Could you check a few things on this model? Use its own coordinates, in mm. A direction names the side the tool comes from. Coordinates: 2 decimals unless noted, no trailing zeros. Order: outer loops, then holes, each group sorted by start corner. A loop starts at its lowest first (then second) coordinate and runs counter-clockwise, first axis right, second up. Notation, with made-up numbers: M 54,-22.75 L 112,-22.75 A23 cw 112,-4.75 Z; hole C 41,17.5 d6. An arc over 180 degrees is marked long. Write item = value, one per line. Start each with the question number.
from build123d import *

# Parameters (mm, degrees)
RESSALTO_EXTRUS_O1_DEPTH          = 10
REBAIXO_PARA_SHCS_M31_D           = 3.4
REBAIXO_PARA_SHCS_M31_CBORE_D     = 6.5
REBAIXO_PARA_SHCS_M31_CBORE_DEPTH = 3
ESBO_O5_W                         = 20.2
ESBO_O5_H                         = 10.9
CORTE_EXTRUS_O1_DEPTH             = 73.325928961
FILETE1_R                         = 5
FILETE2_R                         = 2


with BuildPart() as part:
    # Esboço1 → Ressalto-extrusão1 (new body)
    with BuildSketch(Plane(origin=(0, 0, 0), x_dir=(0, 0, -1), z_dir=(1, 0, 0))):
        Polygon((0, 0), (0, 6), (19.9, 6), (19.9, 15.2), (50.1, 15.2), (50.1, 6), (70, 6), (70, 0), align=None)
    extrude(amount=RESSALTO_EXTRUS_O1_DEPTH)

    # Rebaixo para SHCS M31 (through all)
    with Locations(Plane(origin=(0, 6, 0), x_dir=(1, 0, 0), z_dir=(0, 1, 0))):
        with Locations((5, 5), (5, 65)):
            CounterBoreHole(REBAIXO_PARA_SHCS_M31_D / 2, REBAIXO_PARA_SHCS_M31_CBORE_D / 2, REBAIXO_PARA_SHCS_M31_CBORE_DEPTH)

    # Esboço5 → Corte-extrusão1 (cut, through all)
    with BuildSketch(Plane(origin=(10, 0, 0), x_dir=(0, 0, -1), z_dir=(1, 0, 0))):
        with Locations((35, 5.45)):
            Rectangle(ESBO_O5_W, ESBO_O5_H)
    extrude(amount=-CORTE_EXTRUS_O1_DEPTH, mode=Mode.SUBTRACT)

    # Filete1
    filete1_edges = [part.edges().sort_by_distance(p)[0] for p in [
        (10, 3, 0),
        (0, 3, 0),
        (10, 3, -70),
        (0, 3, -70),
    ]]
    fillet(filete1_edges, radius=FILETE1_R - 0.0001)  # a hair under: the kernel refuses the full size

    # Filete2
    filete2_edges = [part.edges().sort_by_distance(p)[0] for p in [
        (5, 15.2, -19.9),
        (5, 15.2, -50.1),
    ]]
    fillet(filete2_edges, radius=FILETE2_R)


solid = part.part
(1) Thinking about a two-plate mould opening in X: for faces 1 (the flat face through (5, 10, -19.9)), 2 (the cylindrical face through (3.38, 1.48, -65.51)), 3 (the flat face through (0, 11.1, -35.4)), which applies, released by +X, released by -X, zero draft, split by the parting line, or undercut?
(2) Please list where these lines run through material, in increasing order: probe 1 along Z at (x, y) = (5, 1.4); probe 2 along Z at (x, y) = (5, 4.8); probe 3 along X at (y, z) = (2.3, -65). Write a range as from..to.
(3) Imagine slicing it at C-C on x = 9.25. List the corners of the cut face in (y, z) for me.
(4) Imagine slicing it at A-A on y = 5.25. Give the number of separate pieces and of enclosed holes in the cut face, plus the area to 3 significant figures.
(5) Will these pins go through, and if not, where does the flat tip stop? P1, Ø3, axis at x = 7, z = -37.5, coming from the -Y side; P2, Ø3, axis at x = 8, y = 9, coming from the -Z side; P3, Ø2, axis at x = 4, y = 8, coming from the +Z side.
(6) Imagine slicing it at D-D on z = -16.5. List the corners of the cut face in (x, y) for me, plus the area to 3 significant figures.
(7) For faces 4 (the flat face through (5, 5, -45.1)), 5 (the flat face through (5, 10, -50.1)), 6 (the cylindrical face through (8.1, 4.52, -5.98)), 7 (the flat face through (5, 6, -12)), which set-ups out of +Z, -Z, +X, -X, +Y, -Y let a thin tool reach every point of the face, with its end or its side?
Response:
q1.face_1 = zero draft
q1.face_2 = undercut
q1.face_3 = released by -X
q2.probe_1 = -70..-66.7, -63.3..-45.1, -24.9..-6.7, -3.3..0
q2.probe_2 = -70..-68.25, -61.75..-45.1, -24.9..-8.25, -1.75..0
q2.probe_3 = 0..3.3, 6.7..10
q3.outline = M 0,-67.63 L 6,-67.63 L 6,-50.1 L 13.2,-50.1 A2 ccw 15.2,-48.1 L 15.2,-21.9 A2 ccw 13.2,-19.9 L 6,-19.9 L 6,-2.37 L 0,-2.37 L 0,-24.9 L 10.9,-24.9 L 10.9,-45.1 L 0,-45.1 Z
q4.separate_pieces = 2
q4.enclosed_holes = 2
q4.area = 410 mm2
q5.P1 = 10.9
q5.P2 = -50.1
q5.P3 = -19.9
q6.outline = M 0,0 L 10,0 L 10,6 L 0,6 Z
q6.area = 60.0 mm2
q7.face_4 = +X, -X, -Y
q7.face_5 = -Z, +X, -X, +Y
q7.face_6 = +Y
q7.face_7 = +Z, +X, -X, +Y
